Source: CAD feature listing. Evaluate the final solid. Frame: model axes, mm. A direction names the side the tool comes from. Coordinates: 2 decimals unless noted, no trailing zeros. Order: outer loops, then holes, each group sorted by start corner. A loop starts at its lowest first (then second) coordinate and runs counter-clockwise, first axis right, second up.
Autodesk Inventor part; units mm, degrees
ref_plane "YZ Plane" through (0, 0, 0) normal (1, 0, 0) x (0, 1, 0)
ref_plane "XZ Plane" through (0, 0, 0) normal (0, 1, 0) x (-1, 0, 0)
ref_plane "XY Plane" through (0, 0, 0) normal (0, 0, 1) x (1, 0, 0)
sketch "Эскиз1" plane through (0, 0, 0) normal (0, 0, 1) x (1, 0, 0)
  arc A0 (2.5506, 14.7816) -> (2.5506, -14.7816) centre (0, 0) ccw
  line L0 (87.5714, 7.5) -> (150, 7.5)
  line L1 (150, 7.5) -> (150, -7.5)
  line L2 (150, -7.5) -> (87.5714, -7.5)
  arc A1 (2.5506, 14.7816) -> (87.5714, 7.5) centre (87.5714, 507.5) ccw
  arc A2 (87.5714, -7.5) -> (2.5506, -14.7816) centre (87.5714, -507.5) ccw
  point P0 (12.9904, 7.5)
  point P1 (12.9904, -7.5)
  point P2 (12.9904, 7.5)
  point P3 (12.9904, -7.5)
  dimension "d0" = 30
  dimension "d1" = 150
  dimension "d13" = 15
  dimension "d14" = 7.5
  dimension "d19" = 500
extrude "Выдавливание1" add sketch "Эскиз1" along normal blind 5
sketch "Эскиз2" plane through (0, 0, 5) normal (0, 0, 1) x (1, 0, 0)
  arc A0 (2.5506, 14.7816) -> (2.5506, -14.7816) centre (0, 0) ccw
  circle A1 centre (0, 0) radius 5
  point P0 (7.7262, 12.8571)
  point P1 (7.7262, -12.8571)
  dimension "d16" = 10
extrude "Выдавливание2" add sketch "Эскиз2" against normal blind 10
properties part number "Рычаг_2"
Q1. Pin query (flat end, axial travel): P1, Ø4, axis at x = 106.5, z = 1.5, coming from the +Y side; P2, Ø5.5, axis at x = 122, z = 3, coming from the -Y side; P3, Ø5, axis at y = -10.5, z = -1, coming from the -X side. Return the tip coordinate at first contact, or that it passes through.
Solutions:
P1: stops at y = 7.5
P2: stops at y = -7.5
P3: stops at x = -12.55
Q2. Material intervals for line 1 along Z through (x, y) = (31, 6); line 2 along Y through (x, z) = (141.5, 0.5); line 3 along X through (y, z) = (7, 3.25), sorted ascending.
Solutions:
line 1: z = 0 to 5
line 2: y = -7.5 to 7.5
line 3: x = -13.27 to 150
Q3. Section query C-C on z = 2.5. Output: boundary loops of the cut face in (x, y).
Solutions:
outline: (2.55, -14.78) arc R499.99 cw to (87.57, -7.5) - (150, -7.5) - (150, 7.5) - (87.57, 7.5) arc R500.01 cw to (2.55, 14.78) arc R15 ccw (long way) to start
Q4. Set-up query: faces 1 (the flat face through (150, 0, 2)), 2 (the flat face through (119, -7.5, 2)), 3 (the flat face through (118, 7.5, 2)), 4 (the cylindrical face through (-1.08, -4.88, -2.46)). Return all of +Z, -Z, +X, -X, +Y, -Y with unobstructed straight access to the full face (end or side cutting, diameter ignored); none if empty.
Solutions:
face 1: +Z, -Z, +X, +Y, -Y
face 2: +Z, -Z, +X, -Y
face 3: +Z, -Z, +X, +Y
face 4: -Z
Q5. Section query A-A on y = 0. Output: boundary loops of the cut face in (x, z), plus the area to 3 significant figures.
Solutions:
outline: (-15, 0) - (-5, 0) - (-5, -5) - (5, -5) - (5, 0) - (150, 0) - (150, 5) - (-15, 5) - close
area: 875 mm2
Q6. Section query B-B on x = 0. Output: boundary loops of the cut face in (y, z).
Solutions:
outline: (-15, 0) - (-5, 0) - (-5, -5) - (5, -5) - (5, 0) - (15, 0) - (15, 5) - (-15, 5) - close
Q7. Section query D-D on x = 101.5. Output: boundary loops of the cut face in (y, z).
Solutions:
outline: (-7.5, 0) - (7.5, 0) - (7.5, 5) - (-7.5, 5) - close
